```python
from build123d import *

# Parameters (mm, degrees)
SKETCH_1_R          = 4
EXTRUDE_1_DEPTH     = 8
SKETCH_2_R          = 3.5
EXTRUDE_2_DEPTH     = 45
CHAMFER_1_SIZE      = 1.5
CHAMFER_1_SIZE_2    = 2.598076211
SKETCH_3_R          = 2
CUT_EXTRUDE_1_DEPTH = 101
CHAMFER_2_SIZE      = 1
CHAMFER_2_SIZE2     = 2.747477419


with BuildPart() as part:
    # 草图1 → 凸台-拉伸1 (new body)
    with BuildSketch(Plane(origin=(0, 0, 0), x_dir=(1, 0, 0), z_dir=(0, 1, 0))):
        with Locations(Location((0, 0, 0), (0, 0, 270))):
            Circle(SKETCH_1_R)
    extrude(amount=EXTRUDE_1_DEPTH)

    # 草图2 → 凸台-拉伸2 (add)
    with BuildSketch(Plane.XZ):
        with Locations(Location((0, 0, 0), (0, 0, 90))):
            Circle(SKETCH_2_R)
    extrude(amount=EXTRUDE_2_DEPTH)

    # 倒角1
    # the kernel refuses this chamfer: 2.598076211, 1.5 mm, written as the material it adds along each edge
    with BuildSketch(Plane(origin=(0, 0, 0), x_dir=(0, 0, 1), z_dir=(1, 0, 0))) as chamfer_1_piece_1_section:
        Polygon((3.5 + CHAMFER_1_SIZE, 0), (3.5, CHAMFER_1_SIZE_2), (3.5, 0), align=None)
    chamfer_1_piece_1 = revolve(axis=Axis((0, 0, 0), (0, -1, 0)), mode=Mode.PRIVATE)
    chamfer_1_piece_1 = chamfer_1_piece_1 & Plane(origin=(0, -2.194625368, 0), x_dir=(0, 0, 1), z_dir=(0, -1, 0)) * Cylinder(4, 20, mode=Mode.PRIVATE)
    add(chamfer_1_piece_1)

    # 草图3 → 切除-拉伸1 (cut)
    with BuildSketch(Plane.XZ.offset(45)):
        with Locations(Location((0, 0, 0), (0, 0, 270))):
            Circle(SKETCH_3_R)
    extrude(amount=-CUT_EXTRUDE_1_DEPTH, mode=Mode.SUBTRACT)

    # 倒角2
    chamfer_2_edges = [part.edges().sort_by_distance(p)[0] for p in [
        (0, 8, 2),
    ]]
    chamfer_2_side = [part.faces().sort_by_distance(p)[0] for p in [
        (0, 8, -3.886862915),
    ]]
    chamfer(chamfer_2_edges, length=CHAMFER_2_SIZE, length2=CHAMFER_2_SIZE2, reference=chamfer_2_side[0])


solid = part.part
```
Source: CAD feature listing. Evaluate the final solid. Frame: model axes, mm. A direction names the side the tool comes from. Give positions to 0.01 mm unless a question says otherwise; leave off trailing zeros. Order: outer loops, then holes, each group sorted by start corner. A loop starts at its lowest first (then second) coordinate and runs counter-clockwise, first axis right, second up.
(1) Pull-direction query (Z, two-part tool) for faces 3 (the face through (-2, -20, 0)), 4 (the face through (2, -45, 2)), 5 (the face through (1.532, 3.066, 3.695)); classes: +Z half, -Z half, draft (parallel to the pull), parting line (faces both ways), or undercut.
(2) Material intervals for line 1 along X through (y, z) = (-34, 0); line 2 along Z through (x, y) = (-1, -11.5); line 3 along Z through (x, y) = (1.5, -9.5), sorted ascending.
(3) Contact query for flat-ended pins moving along their axis: P1, Ø3, axis at x = -2, y = -36.5, coming from the -Z side; P2, Ø4, axis at y = -18.5, z = -2.5, coming from the -X side; P3, Ø1, axis at y = -15, z = 0.5, coming from the +X side. Output: stop coordinate, or through.
(4) Section query A-A (z = 0). Return the cut outline in (x, y), plus the area to 3 significant figures.
(5) Access query for faces 1 (the face through (3.417, -23.502, -0.759)), 2 (the face through (3, 8, 1)). Directions: +Z, -Z, +X, -X, +Y, -Y. A direction counts if a zero-diameter tool reaches every point of the face in a straight line with its end or side. Return the directions, or none.
(6) Section query C-C (y = -33). Return the cut outline in (x, z), plus the area to 3 significant figures.
(7) Section query B-B (x = 0). Return the cut outline in (y, z), plus the area to 3 significant figures.
Outcome:
1. face 3: undercut
1. face 4: draft
1. face 5: parting line
2. line 1: x = -3.5 to -2, 2 to 3.5
2. line 2: z = -3.35 to -1.73, 1.73 to 3.35
2. line 3: z = -3.16 to -1.32, 1.32 to 3.16
3. P1: stops at z = -3.46
3. P2: stops at x = -3.46
3. P3: stops at x = 3.5
4. outline: (-4, -1.73) - (-3.5, -2.6) - (-3.5, -45) - (-2, -45) - (-2, 5.25) - (-3, 8) - (-4, 8) - close; (2, -45) - (3.5, -45) - (3.5, -2.6) - (4, -1.73) - (4, 8) - (3, 8) - (2, 5.25) - close
4. area: 166 mm2
5. face 1: -Y
5. face 2: +Z, -Z, +X, -X, +Y
6. outline: circle Ø7 at (0, 0); hole circle Ø4 at (0, 0)
6. area: 25.9 mm2
7. outline: (-45, -3.5) - (-2.6, -3.5) - (-1.73, -4) - (8, -4) - (8, -3) - (5.25, -2) - (-45, -2) - close; (-45, 2) - (5.25, 2) - (8, 3) - (8, 4) - (-1.73, 4) - (-2.6, 3.5) - (-45, 3.5) - close
7. area: 166 mm2
